CAD build for the part. Positions are in the model's coordinates, mm. Round coordinates to 2 decimals unless told otherwise and drop trailing zeros. Loops run counter-clockwise (first coordinate to the right, second up) from the corner with the lowest first, then second, coordinate; pieces in that order, holes last.
from build123d import *

# Parameters (mm, degrees)
SKETCH1_W               = 575
SKETCH1_H               = 120
BOSS_EXTRUDE1_DEPTH     = 1.5875
M3_CLEARANCE_HOLE1_D    = 3.4
F_3_8_CLEARANCE_HOLE1_D = 10.0838
LPATTERN1_COUNT         = 13
LPATTERN1_PITCH         = 30
CUT_EXTRUDE1_REACH      = 295.698
SKETCH8_R               = 1.95
SKETCH8_R_2             = 1.2
CUT_EXTRUDE2_REACH      = 295.698
SKETCH9_W               = 28
SKETCH9_H               = 20
FILLET1_R               = 4
CHAMFER1_SIZE           = 5
CUT_EXTRUDE3_REACH      = 295.698
SKETCH10_R              = 6


with BuildPart() as part:
    # Sketch1 → Boss-Extrude1 (new body)
    with BuildSketch(Plane.XY):
        Rectangle(SKETCH1_W, SKETCH1_H)
    extrude(amount=BOSS_EXTRUDE1_DEPTH)

    # M3 Clearance Hole1 (through all)
    with Locations(Plane.XY.offset(1.5875)):
        with Locations((-257.5, -25), (-217.5, -25)):
            Hole(M3_CLEARANCE_HOLE1_D / 2)

    # 3/8 Clearance Hole1 (through all)
    with Locations(Plane.XY.offset(1.5875)):
        with Locations((-117.5, 0)):
            f_3_8_clearance_hole1 = Hole(F_3_8_CLEARANCE_HOLE1_D / 2)

    # LPattern1: 3/8 Clearance Hole1 ×13
    with Locations(*[(i * LPATTERN1_PITCH, 0, 0) for i in range(1, LPATTERN1_COUNT)]):
        add(f_3_8_clearance_hole1, mode=Mode.SUBTRACT)

    # Sketch8 → Cut-Extrude1 (cut, up to next)
    with BuildSketch(Plane.XY.offset(1.5875), mode=Mode.PRIVATE) as cut_extrude1_sk1:
        with Locations((-187.5, 30)):
            Circle(SKETCH8_R)
    cut_extrude1_tool1 = extrude(cut_extrude1_sk1.sketch, amount=-CUT_EXTRUDE1_REACH, mode=Mode.PRIVATE) & part.part
    # Sketch8 → Cut-Extrude1 (cut, up to next)
    with BuildSketch(Plane.XY.offset(1.5875), mode=Mode.PRIVATE) as cut_extrude1_sk2:
        with Locations((-170.99, 30)):
            Circle(SKETCH8_R_2)
    cut_extrude1_tool2 = extrude(cut_extrude1_sk2.sketch, amount=-CUT_EXTRUDE1_REACH, mode=Mode.PRIVATE) & part.part
    add(cut_extrude1_tool1.solids().sort_by_distance((-187.5, 30, 1.5875))[0], mode=Mode.SUBTRACT)
    add(cut_extrude1_tool2.solids().sort_by_distance((-170.99, 30, 1.5875))[0], mode=Mode.SUBTRACT)

    # Sketch9 → Cut-Extrude2 (cut, up to next)
    with BuildSketch(Plane.XY.offset(1.5875), mode=Mode.PRIVATE) as cut_extrude2_sk1:
        with Locations((-237.5, -25)):
            Rectangle(SKETCH9_W, SKETCH9_H)
    cut_extrude2_tool1 = extrude(cut_extrude2_sk1.sketch, amount=-CUT_EXTRUDE2_REACH, mode=Mode.PRIVATE) & part.part
    add(cut_extrude2_tool1.solids().sort_by_distance((-237.5, -25, 1.5875))[0], mode=Mode.SUBTRACT)

    # Fillet1
    fillet1_edges = [part.edges().sort_by_distance(p)[0] for p in [
        (-251.5, -35, 0.79375),
        (-223.5, -35, 0.79375),
    ]]
    fillet(fillet1_edges, radius=FILLET1_R)

    # Chamfer1
    chamfer1_edges = [part.edges().sort_by_distance(p)[0] for p in [
        (-251.5, -15, 0.79375),
        (-223.5, -15, 0.79375),
    ]]
    chamfer(chamfer1_edges, length=CHAMFER1_SIZE)

    # Sketch10 → Cut-Extrude3 (cut, up to next)
    with BuildSketch(Plane.XY.offset(1.5875), mode=Mode.PRIVATE) as cut_extrude3_sk1:
        with Locations((-237.5, 20)):
            Circle(SKETCH10_R)
    cut_extrude3_tool1 = extrude(cut_extrude3_sk1.sketch, amount=-CUT_EXTRUDE3_REACH, mode=Mode.PRIVATE) & part.part
    add(cut_extrude3_tool1.solids().sort_by_distance((-237.5, 20, 1.5875))[0], mode=Mode.SUBTRACT)


solid = part.part
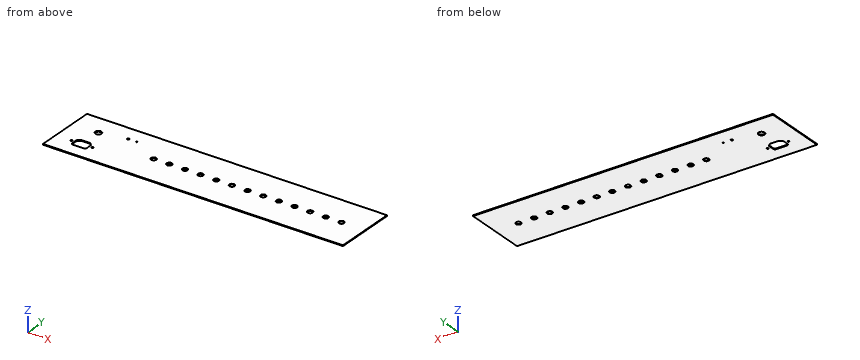
Item 1: Flat gauge pins, fed straight in: P1, Ø13, axis at x = -117.5, y = 0, coming from the -Z side; P2, Ø6, axis at x = 212.5, y = 0, coming from the -Z side. Where does each tip first touch, or does it go through?
Verdict:
P1: stops at z = 0
P2: passes through
Item 2: Cut at A-A (x = 182.5). List the corners of the cut face in (y, z).
Verdict:
outline: (-60, 0) - (-5.04, 0) - (-5.04, 1.59) - (-60, 1.59) - close; (5.04, 0) - (60, 0) - (60, 1.59) - (5.04, 1.59) - close
Item 3: Wall check: L1, parallel to Y at x = 2.5, z = 0.4; L2, parallel to Y at x = -217.5, z = 0.9; L3, parallel to X at y = 14.5, z = 0.8. Give the ranges that are in metal, low to high.
Verdict:
L1: y = -60 to -5.04, 5.04 to 60
L2: y = -60 to -26.7, -23.3 to 60
L3: x = -287.5 to -239.9, -235.1 to 287.5
Item 4: Cut at B-B (z = 1.2). State how many separate pieces and enclosed holes the cut face has, plus the area to 3 significant figures.
Verdict:
separate pieces: 1
enclosed holes: 19
area: 67,300 mm2
